from build123d import *

# Parameters (mm, degrees)
F0_W     = 100
F0_H     = 50
F1_DEPTH = 15
F2_W     = 5
F2_H     = 5
F3_DEPTH = 8.5
F4_DEPTH = 15.001
F5_W     = 28
F5_H     = 48
F5_W_2   = 5
F5_H_2   = 5
F5_W_3   = 29
F6_DEPTH = 14
F5_W_4   = 42
F7_DEPTH = 5.5
F8_R     = 9
F9_R     = 10


with BuildPart() as f1:
    # F0 (on Top) → F1 (new body)
    with BuildSketch(Plane.XY):
        with Locations((-50, 25)):
            Rectangle(F0_W, F0_H)
    extrude(amount=F1_DEPTH)

    # F2 (on face) → F3 (cut)
    with BuildSketch(Plane.XY.offset(15)):
        Polygon((-30, 45), (-30, 50), (-70, 50), (-70, 0), (-30, 0), align=None)
        with Locations((-57.5, 12.5)):
            Rectangle(F2_W, F2_H, mode=Mode.SUBTRACT)
        with Locations((-37.5, 12.5)):
            Rectangle(F2_W, F2_H, mode=Mode.SUBTRACT)
        with Locations((-57.5, 42.5)):
            Rectangle(F2_W, F2_H, mode=Mode.SUBTRACT)
        with Locations((-37.5, 42.5)):
            Rectangle(F2_W, F2_H, mode=Mode.SUBTRACT)
    extrude(amount=-F3_DEPTH, mode=Mode.SUBTRACT)

    # F2 (on face) → F4 (cut, through all)
    with BuildSketch(Plane.XY.offset(15)):
        with Locations((-77.5, 42.5)):
            Rectangle(F2_W, F2_H)
        with Locations((-77.5, 27.5)):
            Rectangle(F2_W, F2_H)
        with Locations((-77.5, 12.5)):
            Rectangle(F2_W, F2_H)
        with Locations((-57.5, 12.5)):
            Rectangle(F2_W, F2_H)
        with Locations((-57.5, 42.5)):
            Rectangle(F2_W, F2_H)
        with Locations((-37.5, 42.5)):
            Rectangle(F2_W, F2_H)
        with Locations((-37.5, 12.5)):
            Rectangle(F2_W, F2_H)
        with Locations((-17.5, 12.5)):
            Rectangle(F2_W, F2_H)
        with Locations((-17.5, 27.5)):
            Rectangle(F2_W, F2_H)
        with Locations((-17.5, 42.5)):
            Rectangle(F2_W, F2_H)
    extrude(amount=-F4_DEPTH, mode=Mode.SUBTRACT)

    # F5 (on face) → F6 (cut)
    with BuildSketch(Plane(origin=(0, 0, 0), x_dir=(1, 0, 0), z_dir=(0, 0, -1))):
        with Locations((-15, -25)):
            Rectangle(F5_W, F5_H)
        with Locations((-17.5, -42.5)):
            Rectangle(F5_W_2, F5_H_2, mode=Mode.SUBTRACT)
        with Locations((-17.5, -27.5)):
            Rectangle(F5_W_2, F5_H_2, mode=Mode.SUBTRACT)
        with Locations((-17.5, -12.5)):
            Rectangle(F5_W_2, F5_H_2, mode=Mode.SUBTRACT)
        with Locations((-85.5, -25)):
            Rectangle(F5_W_3, F5_H)
        with Locations((-77.5, -42.5)):
            Rectangle(F5_W_2, F5_H_2, mode=Mode.SUBTRACT)
        with Locations((-77.5, -27.5)):
            Rectangle(F5_W_2, F5_H_2, mode=Mode.SUBTRACT)
        with Locations((-77.5, -12.5)):
            Rectangle(F5_W_2, F5_H_2, mode=Mode.SUBTRACT)
    extrude(amount=-F6_DEPTH, mode=Mode.SUBTRACT)

    # F5 (on face) → F7 (cut)
    with BuildSketch(Plane(origin=(0, 0, 0), x_dir=(1, 0, 0), z_dir=(0, 0, -1))):
        with Locations((-50, -25)):
            Rectangle(F5_W_4, F5_H)
        with Locations((-57.5, -42.5)):
            Rectangle(F5_W_2, F5_H_2, mode=Mode.SUBTRACT)
        with Locations((-37.5, -42.5)):
            Rectangle(F5_W_2, F5_H_2, mode=Mode.SUBTRACT)
        with Locations((-57.5, -12.5)):
            Rectangle(F5_W_2, F5_H_2, mode=Mode.SUBTRACT)
        with Locations((-37.5, -12.5)):
            Rectangle(F5_W_2, F5_H_2, mode=Mode.SUBTRACT)
    extrude(amount=-F7_DEPTH, mode=Mode.SUBTRACT)

    # F8
    f8_edges = [f1.edges().sort_by_distance(p)[0] for p in [
        (-1, 49, 7),
        (-1, 1, 7),
    ]]
    fillet(f8_edges, radius=F8_R)

    # F9
    f9_edges = [f1.edges().sort_by_distance(p)[0] for p in [
        (0, 50, 7.5),
        (0, 0, 7.5),
    ]]
    fillet(f9_edges, radius=F9_R)


solid = f1.part
Input: part model. Units: mm. Frame: model coordinates. A direction names the side the tool comes from. Coordinates: 2 decimals unless noted, no trailing zeros. Loops run counter-clockwise (first coordinate to the right, second up) from the corner with the lowest first, then second, coordinate; pieces in that order, holes last. Notation, with made-up numbers: (41, 89) -> (58, 89) arc R34 ccw to (58, 121) -> close; hole circle Ø9 at (70.25, -40). An arc over 180 degrees is marked (long way). One line per item, written item: value.
(1) Cut plane C-C (z = 9). Output: boundary loops of the cut face in (x, y), then the cut area to 3 significant figures.
Answer below:
outline: (-100, 0) -> (-70, 0) -> (-70, 50) -> (-100, 50) -> (-100, 49) -> (-71, 49) -> (-71, 1) -> (-100, 1) -> close; (-30, 0) -> (-10, 0) arc R10 ccw to (0, 10) -> (0, 40) arc R10 ccw to (-10, 50) -> (-30, 50) -> close; hole (-29, 1) -> (-10, 1) arc R9 ccw to (-1, 10) -> (-1, 40) arc R9 ccw to (-10, 49) -> (-29, 49) -> close
area: 256 mm2
(2) Draft query along Y for faces 4 (the face through (-29, 25, 10)), 5 (the face through (0, 25, 7)), 6 (the face through (-56, 0, 6)). Return one class per face: pulls with the +Y half, pulls with the -Y half, needs draft (parallel to the pull), parting line crosses it, or undercut.
Answer below:
face 4: undercut
face 5: needs draft
face 6: pulls with the -Y half
(3) Ray query, line 1 along X through (y, z) = (11.5, 12.75); line 2 along X through (y, z) = (46, 12.75); line 3 along Y through (x, z) = (-88.5, 12). Return the intervals inside material, ascending.
Answer below:
line 1: x = -71 to -70, -30 to -29, -1 to 0
line 2: x = -71 to -70, -30 to -29, -3.29 to -2
line 3: y = 0 to 1, 49 to 50
(4) Pin query (flat end, axial travel): pin 1 Ø1 at (x, y) = (-55, 32.5) entering from +Z; pin 2 Ø1.1 at (y, z) = (42, 6) entering from -X; pin 3 Ø8.5 at (x, y) = (-90.5, 29) entering from -Z. Return the tip coordinate at first contact, or that it passes through.
Answer below:
pin 1: stops at z = 6.5
pin 2: stops at x = -71
pin 3: stops at z = 14
(5) Cut plane A-A (y = 26.5). Output: boundary loops of the cut face in (x, z).
Answer below:
outline: (-100, 14) -> (-80, 14) -> (-80, 15) -> (-100, 15) -> close; (-75, 14) -> (-71, 14) -> (-71, 5.5) -> (-29, 5.5) -> (-29, 14) -> (-20, 14) -> (-20, 15) -> (-30, 15) -> (-30, 6.5) -> (-70, 6.5) -> (-70, 15) -> (-75, 15) -> close; (-15, 14) -> (-1, 14) -> (-1, 0) -> (0, 0) -> (0, 15) -> (-15, 15) -> close
(6) Cut plane B-B (x = -16.5). Output: boundary loops of the cut face in (y, z), then the cut area to 3 significant figures.
Answer below:
outline: (0, 0) -> (1, 0) -> (1, 14) -> (10, 14) -> (10, 15) -> (0, 15) -> close; (15, 14) -> (25, 14) -> (25, 15) -> (15, 15) -> close; (30, 14) -> (40, 14) -> (40, 15) -> (30, 15) -> close; (45, 14) -> (49, 14) -> (49, 0) -> (50, 0) -> (50, 15) -> (45, 15) -> close
area: 63.0 mm2
(7) Cut plane D-D (x = -58). Output: boundary loops of the cut face in (y, z), then the cut area to 3 significant figures.
Answer below:
outline: (0, 0) -> (1, 0) -> (1, 5.5) -> (10, 5.5) -> (10, 6.5) -> (0, 6.5) -> close; (15, 5.5) -> (40, 5.5) -> (40, 6.5) -> (15, 6.5) -> close; (45, 5.5) -> (49, 5.5) -> (49, 0) -> (50, 0) -> (50, 6.5) -> (45, 6.5) -> close
area: 51.0 mm2
(8) Set-up query: faces 1 (the face through (-3.566, 3.706, 7.098)), 2 (the face through (-86, 25, 14)), 3 (the face through (-30, 25, 11)). Return all of +Z, -Z, +X, -X, +Y, -Y with unobstructed straight access to the full face (end or side cutting, diameter ignored); none if empty.
Answer below:
face 1: -Z
face 2: -Z, -X
face 3: +Z, +Y, -Y
